Build history of the part. All positions in model axes, mm. A direction names the side the tool comes from. Round coordinates to 2 decimals unless told otherwise and drop trailing zeros. Write each loop counter-clockwise with the first axis right and the second up, starting at its lowest first coordinate (ties: lowest second). Pieces come first, ordered by that corner, then holes. Notation, with made-up numbers: (2, 6) -> (17, 6) arc R31 cw to (17, 33) -> close; hole circle Ø7 at (62.5, 56). An arc over 180 degrees is marked (long way). Answer in a Markdown table with one row per item. Add a question column.
from build123d import *

# Parameters (mm, degrees)
F0_R     = 3.25
F0_R_2   = 10
F1_DEPTH = 10
F2_R     = 22
F2_R_2   = 10
F3_DEPTH = 6
F4_R     = 16
F4_R_2   = 10
F5_DEPTH = 9
F6_R     = 22
F6_R_2   = 10
F7_DEPTH = 14
F8_R     = 16
F8_R_2   = 10
F9_DEPTH = 9
F10_SIZE = 0.5


with BuildPart() as f1:
    # F0 (on Top) → F1 (new body)
    with BuildSketch(Plane.XY):
        with BuildLine():
            Line((-21.6506350946, -27.5), (21.6506350946, -27.5))
            ThreePointArc((21.6506350946, -27.5), (0, 35), (-21.6506350946, -27.5))
        make_face()
        with Locations((-25, -15)):
            Circle(F0_R, mode=Mode.SUBTRACT)
        with Locations((25, -15)):
            Circle(F0_R, mode=Mode.SUBTRACT)
        Circle(F0_R_2, mode=Mode.SUBTRACT)
        with Locations((-25, 15)):
            Circle(F0_R, mode=Mode.SUBTRACT)
        with Locations((25, 15)):
            Circle(F0_R, mode=Mode.SUBTRACT)
    extrude(amount=F1_DEPTH)

    # F2 (on face) → F3 (join)
    with BuildSketch(Plane.XY.offset(10)):
        Circle(F2_R)
        Circle(F2_R_2, mode=Mode.SUBTRACT)
    extrude(amount=F3_DEPTH)

    # F4 (on face) → F5 (cut)
    with BuildSketch(Plane.XY.offset(16)):
        Circle(F4_R)
        Circle(F4_R_2, mode=Mode.SUBTRACT)
    extrude(amount=-F5_DEPTH, mode=Mode.SUBTRACT)

    # F6 (on face) → F7 (join)
    with BuildSketch(Plane(origin=(0, 0, 0), x_dir=(1, 0, 0), z_dir=(0, 0, -1))):
        Circle(F6_R)
        Circle(F6_R_2, mode=Mode.SUBTRACT)
    extrude(amount=F7_DEPTH)

    # F8 (on face) → F9 (cut)
    with BuildSketch(Plane(origin=(0, 0, -14), x_dir=(1, 0, 0), z_dir=(0, 0, -1))):
        Circle(F8_R)
        Circle(F8_R_2, mode=Mode.SUBTRACT)
    extrude(amount=-F9_DEPTH, mode=Mode.SUBTRACT)

    # F10
    f10_edges = [f1.edges().sort_by_distance(p)[0] for p in [
        (-28.25, -15, 10),
        (-28.25, 15, 10),
        (21.75, 15, 10),
        (21.75, -15, 10),
        (21.75, 15, 0),
        (21.75, -15, 0),
        (-28.25, 15, 0),
        (-28.25, -15, 0),
    ]]
    chamfer(f10_edges, length=F10_SIZE)


solid = f1.part
(1) Drop flat-ended pins along their axis: P1, Ø23, axis at x = 0, y = 0, coming from the -Z side; P2, Ø2, axis at y = 1.5, z = 7, coming from the +X side; P3, Ø4, axis at y = 9.5, z = 10.5, coming from the -X side. Give the stop position or say it passes through.
(2) Saw through at C-C (x = 25). List the corners of the cut face in (y, z).
(3) Probe line 1 along Y through (x, z) = (0, -8); line 2 along Y through (x, z) = (-25, 5.5). List the from-to ranges inside material, lowest first.
(4) Saw through at B-B (y = 0). List the corners of the cut face in (x, z), plus the area to 3 significant figures.
(5) Saw through at A-A (x = 0). List the corners of the cut face in (y, z).
(6) Saw through at D-D (z = 3). List the corners of the cut face in (x, y), plus the area to 3 significant figures.
(7) Which spindle directions (+Z, -Z, +X, -X, +Y, -Y) get a long thin tool onto all of the face, cutting with end or side? Do faces 1 (the face through (-4.769, -21.477, 12.958)), 2 (the face through (-2.17, 9.76, 1.08)), 3 (the face through (-3.47, 15.62, -9.56)). Say none if no direction does.
(8) Mould opens along X. For faces 4 (the face through (15, 18, 0)), 5 (the face through (10.4, 0.2, 7)), 6 (the face through (-4.769, 21.477, -6.902)) say: pulls with the +X half, pulls with the -X half, needs draft (parallel to the pull), parting line crosses it, or undercut.
Answer sheet:
| question | item | result |
|---|---|---|
| 1 | P1 | stops at z = -5 |
| 1 | P2 | stops at x = 35 |
| 1 | P3 | stops at x = -34.17 |
| 2 | outline | (-24.49, 0) -> (-18.75, 0) -> (-18.25, 0.5) -> (-18.25, 9.5) -> (-18.75, 10) -> (-24.49, 10) -> close; (-11.75, 0.5) -> (-11.25, 0) -> (11.25, 0) -> (11.75, 0.5) -> (11.75, 9.5) -> (11.25, 10) -> (-11.25, 10) -> (-11.75, 9.5) -> close; (18.25, 0.5) -> (18.75, 0) -> (24.49, 0) -> (24.49, 10) -> (18.75, 10) -> (18.25, 9.5) -> close |
| 3 | line 1 | y = -22 to -16, 16 to 22 |
| 3 | line 2 | y = -24.49 to -18.25, -11.75 to 11.75, 18.25 to 24.49 |
| 4 | outline | (-35, 0) -> (-22, 0) -> (-22, -14) -> (-16, -14) -> (-16, -5) -> (-10, -5) -> (-10, 7) -> (-16, 7) -> (-16, 16) -> (-22, 16) -> (-22, 10) -> (-35, 10) -> close; (10, -5) -> (16, -5) -> (16, -14) -> (22, -14) -> (22, 0) -> (35, 0) -> (35, 10) -> (22, 10) -> (22, 16) -> (16, 16) -> (16, 7) -> (10, 7) -> close |
| 4 | area | 764 mm² |
| 5 | outline | (-27.5, 0) -> (-22, 0) -> (-22, -14) -> (-16, -14) -> (-16, -5) -> (-10, -5) -> (-10, 7) -> (-16, 7) -> (-16, 16) -> (-22, 16) -> (-22, 10) -> (-27.5, 10) -> close; (10, -5) -> (16, -5) -> (16, -14) -> (22, -14) -> (22, 0) -> (35, 0) -> (35, 10) -> (22, 10) -> (22, 16) -> (16, 16) -> (16, 7) -> (10, 7) -> close |
| 6 | outline | (-21.65, -27.5) -> (21.65, -27.5) arc R35 ccw (long way) to start; hole circle Ø6.5 at (-25, -15); hole circle Ø6.5 at (-25, 15); hole circle Ø20 at (0, 0); hole circle Ø6.5 at (25, -15); hole circle Ø6.5 at (25, 15) |
| 6 | area | 3,180 mm² |
| 7 | face 1 | +Z |
| 7 | face 2 | +Z, -Z |
| 7 | face 3 | -Z |
| 8 | face 4 | needs draft |
| 8 | face 5 | undercut |
| 8 | face 6 | parting line crosses it |
